```python
from build123d import *

# Parameters (mm, degrees)
MAIN_DEPTH                   = 85
BACKBRACKETHOLES_D           = 4.572
BACKBRACKETHOLES_DEPTH       = 5
BACKBRACKETHOLES_CSINK_D     = 7.9248
BACKBRACKETHOLES_CSINK_ANGLE = 82
FRONT_CUT_REACH              = 115.044


with BuildPart() as part:
    # Sketch1 → Main (new, symmetric)
    with BuildSketch(Plane(origin=(0, 0, 0), x_dir=(0, 0, -1), z_dir=(1, 0, 0))):
        Polygon((0, 0), (-2.3622, 0), (23.115716399, 70), (25.477916399, 70), align=None)
    extrude(amount=MAIN_DEPTH, both=True)

    # BackBracketHoles
    with Locations(Plane(origin=(0, 0.759196446, 2.085875092), x_dir=(1, 0, 0), z_dir=(0, 0.3420201433256726, 0.9396926207859071))):
        with Locations((-67.6378, 50.002080017), (-47.6378, 25.002080017)):
            CounterSinkHole(BACKBRACKETHOLES_D / 2, BACKBRACKETHOLES_CSINK_D / 2, depth=BACKBRACKETHOLES_DEPTH, counter_sink_angle=BACKBRACKETHOLES_CSINK_ANGLE)

    # Sketch4 → Front Cut (cut, up to next)
    with BuildSketch(Plane(origin=(0, 0.759196446, 2.085875092), x_dir=(1, 0, 0), z_dir=(0, 0.3420201433256726, 0.9396926207859071)), mode=Mode.PRIVATE) as front_cut_sk1:
        Polygon((85, -0.807919983), (9.699635944, 74.492444073), (85, 74.492444073), align=None)
    front_cut_tool1 = extrude(front_cut_sk1.sketch, amount=-FRONT_CUT_REACH, mode=Mode.PRIVATE) & part.part
    add(front_cut_tool1.solids().sort_by_distance((59.899879, 47.172798, -14.807294))[0], mode=Mode.SUBTRACT)


solid = part.part
```
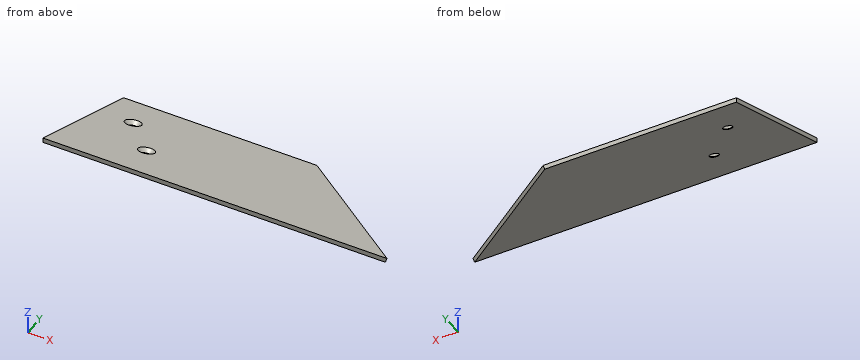
Verification items for the finished model (mm, model axes). Round coordinates to 2 decimals unless told otherwise and drop trailing zeros. Order: outer loops, then holes, each group sorted by start corner. A loop starts at its lowest first (then second) coordinate and runs counter-clockwise, first axis right, second up. Notation, with made-up numbers: (36, 4) - (80, 4) arc R21 cw to (80, 30) - close; hole circle Ø4 at (-36.75, -3.5). An arc over 180 degrees is marked (long way). Use CSV: the item, a comma, the result in double quotes.
(1) Section check B-B on z = -20. Record the boundary of the cut face in (x, y).
Entries:
outline,"(-85, 54.95) - (25.72, 54.95) - (19.62, 61.44) - (-85, 61.44) - close"
(2) Section check A-A on x = -33.5. Record the boundary of the cut face in (y, z), and give its area (3 significant figures).
Entries:
outline,"(0, 0) - (70, -25.48) - (70, -23.12) - (0, 2.36) - close"
area,"165 mm^2"
(3) Thickness scan on probe 1 along Z at (x, y) = (-75, 44); probe 2 along Z at (x, y) = (8.5, 11.5); probe 3 along X at (y, z) = (59.5, -20.75). Record the ranges inside material, lowest first. Write a range as from..to.
Entries:
probe 1,"-16.01..-13.65"
probe 2,"-4.19..-1.82"
probe 3,"-85..21.18"
(4) Gauge pin test, flat ends, axial feed: pin 1 Ø1.5 at (x, z) = (49.5, -11) entering from +Y; pin 2 Ø8 at (x, y) = (27, 32) entering from +Z; pin 3 Ø4 at (x, y) = (-19.5, 40) entering from -Z. Record the tip position at first contact, or that the pin passes through.
Entries:
pin 1,"y = 33.76"
pin 2,"z = -7.83"
pin 3,"z = -15.29"
